The model under review builds one solid part; all positions refer to its coordinate system, in mm. Face numbers are marked on the shaded views. A direction names the side the tool comes from. Coordinates: 2 decimals unless noted, no trailing zeros. Order: outer loops, then holes, each group sorted by start corner. A loop starts at its lowest first (then second) coordinate and runs counter-clockwise, first axis right, second up. Notation, with made-up numbers: M 33.5,29 L 72.5,29 A11 cw 72.5,37 Z; hole C 72,13 d7. An arc over 180 degrees is marked long. Answer in a Markdown table with one row per item.
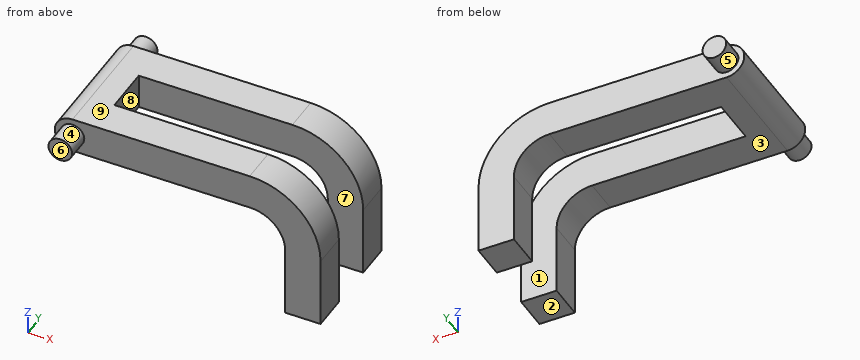
from build123d import *

# Parameters (mm, degrees)
EXTRUDE_1_DEPTH      = 42.498268572
EXTRUDE_1_DEPTH_BACK = 7.5
SKETCH_1_R           = 5
SKETCH_2_R           = 5
EXTRUDE_2_DEPTH      = 17.5
SKETCH_3_R           = 5
EXTRUDE_3_DEPTH      = 52.5
SKETCH_4_W           = 107.730205786
SKETCH_4_H           = 74.358975683
CUT_EXTRUDE_1_DEPTH  = 10


with BuildPart() as part:
    # 草图1 → 凸台-拉伸1 (new, two sides: drawn at the far end of the back side and taken through both)
    with BuildSketch(Plane(origin=(0, 0, 0), x_dir=(1, 0, 0), z_dir=(0, 1, 0)).offset(-EXTRUDE_1_DEPTH_BACK)):
        with BuildLine():
            Line((0, 0), (75, 0))
            ThreePointArc((75, 0), (96.213203436, 8.786796564), (105, 30))
            Line((105, 30), (105, 60))
            Line((105, 60), (90, 60))
            Line((90, 60), (90, 30))
            ThreePointArc((90, 30), (85.606601718, 19.393398282), (75, 15))
            Line((75, 15), (0, 15))
            ThreePointArc((0, 15), (-7.5, 7.5), (0, 0))
        make_face()
        with Locations(Location((0, 7.5, 0), (0, 0, 270))):
            Circle(SKETCH_1_R, mode=Mode.SUBTRACT)
    extrude(amount=EXTRUDE_1_DEPTH + EXTRUDE_1_DEPTH_BACK)

    # 草图2 → 凸台-拉伸2 (add, symmetric)
    with BuildSketch(Plane(origin=(0, 0, 0), x_dir=(1, 0, 0), z_dir=(0, 1, 0))):
        with Locations(Location((0, 7.5, 0), (0, 0, 270))):
            Circle(SKETCH_2_R)
    extrude(amount=EXTRUDE_2_DEPTH, both=True)

    # 草图3 → 凸台-拉伸3 (add)
    with BuildSketch(Plane(origin=(0, 0, 0), x_dir=(1, 0, 0), z_dir=(0, 1, 0))):
        with Locations(Location((0, 7.5, 0), (0, 0, 270))):
            Circle(SKETCH_3_R)
    extrude(amount=EXTRUDE_3_DEPTH)

    # 草图4 → 切除-拉伸1 (cut, symmetric)
    with BuildSketch(Plane(origin=(0, 17.5, 0), x_dir=(1, 0, 0), z_dir=(0, 1, 0))):
        with Locations((63.865102893, 35.82913053)):
            Rectangle(SKETCH_4_W, SKETCH_4_H)
    extrude(amount=CUT_EXTRUDE_1_DEPTH, both=True, mode=Mode.SUBTRACT)


solid = part.part
(1) To check wall thickness, follow line 1 (Y direction, x = 50, z = -5.5); line 2 (Z direction, x = 39, y = 29.5); line 3 (X direction, y = 36.5, z = -54.5). State the ranges of each line that lie inside material, in increasing order. Write a range as [from, to].
Report:
| item | result |
|---|---|
| line 1 | [-7.5, 7.5], [27.5, 42.5] |
| line 2 | [-15, 0] |
| line 3 | [90, 105] |
(2) Take a section at D-D (z = -7.5). Write out the cut boundary in (x, y).
Report:
| item | result |
|---|---|
| outline | M -7.5,-7.5 L -5,-7.5 L -5,-17.5 L 5,-17.5 L 5,-7.5 L 94.84,-7.5 L 94.84,7.5 L 10,7.5 L 10,27.5 L 94.84,27.5 L 94.84,42.5 L 5,42.5 L 5,52.5 L -5,52.5 L -5,42.5 L -7.5,42.5 Z |
(3) Machinability: for the marked faces 1, 2, 3, 4 and 5, which of the approach directions +Z, -Z, +X, -X, +Y, -Y give a long, thin tool a straight path to every point of the face, cutting with its end or side? Answer none if there is none.
Report:
| item | result |
|---|---|
| face 1 | +Z, -Z, +X |
| face 2 | -Z, +X, -X, +Y, -Y |
| face 3 | -Z, -X, +Y, -Y |
| face 4 | -Y |
| face 5 | +Y |
(4) Take a section at A-A (x = 39.5). Write out the cut boundary in (y, z), then the cut area to 3 significant figures.
Report:
| item | result |
|---|---|
| outline | M -7.5,-15 L 7.5,-15 L 7.5,0 L -7.5,0 Z; M 27.5,-15 L 42.5,-15 L 42.5,0 L 27.5,0 Z |
| area | 450 mm^2 |
(5) Take a section at C-C (y = 39). Write out the cut boundary in (x, z).
Report:
| item | result |
|---|---|
| outline | M 0,-15 L 75,-15 A15 cw 90,-30 L 90,-60 L 105,-60 L 105,-30 A30 ccw 75,0 L 0,0 A7.5 ccw Z |
(6) Take a section at B-B (z = -48.5). Write out the cut boundary in (x, y).
Report:
| item | result |
|---|---|
| outline | M 90,-7.5 L 105,-7.5 L 105,7.5 L 90,7.5 Z; M 90,27.5 L 105,27.5 L 105,42.5 L 90,42.5 Z |
(7) Insertion check: P1, Ø1.5, axis at y = 2, z = -12, coming from the +X side; P2, Ø7.5, axis at y = 2, z = -39, coming from the -X side; P3, Ø1.5, axis at x = 76, z = -7, coming from the +Y side. Each pin has a flat end and moves straight along its axis. Give the tip position at first contact, or say it passes through.
Report:
| item | result |
|---|---|
| P1 | x = 99.54 |
| P2 | x = 90 |
| P3 | y = 42.5 |
(8) The part is to be moulded in two halves that separate along Y. For the marked faces 6, 7, 8 and 9, say which applies: +Y half, -Y half, draft (parallel to the pull), parting line (faces both ways), or undercut.
Report:
| item | result |
|---|---|
| face 6 | -Y half |
| face 7 | undercut |
| face 8 | undercut |
| face 9 | draft |
